Geometry check sheet. Reference: the model listing, model coordinates, mm. Face numbers are marked on the shaded views. A direction names the side the tool comes from. Coordinates: 2 decimals unless noted, no trailing zeros. Write each loop counter-clockwise with the first axis right and the second up, starting at its lowest first coordinate (ties: lowest second). Pieces come first, ordered by that corner, then holes. Notation, with made-up numbers: (56.25, 68) -> (65.25, 68) arc R31 cw to (65.25, 105) -> close; hole circle Ø10 at (74.25, -12.5). An arc over 180 degrees is marked (long way). Answer in a Markdown table with one row per item. Add a question column.
1. Set-up check for the marked faces 1 and 2: record each of +Z, -Z, +X, -X, +Y, -Y from which the full face is reachable in a straight line by a thin tool's end or side.
2. Cross-section at B-B on z = 41. Record the cut outline in (x, y).
3. Scan lines: L1, parallel to Z at x = 3, y = 14; L2, parallel to Z at x = -13, y = -12.5; L3, parallel to Y at x = -4.5, z = 51. Record each from-to range of solid material in increasing order. Write a range as from..to.
4. Mould release check, pull along X, two halves, no side actions. Record for the marked faces 3, 4 and 5: pulls with the +X half, pulls with the -X half, needs draft (parallel to the pull), parting line crosses it, or undercut.
5. Depth check by flat-ended pin: P1, Ø2, axis at y = 11.5, z = 16.5, coming from the -X side; P2, Ø3, axis at x = 3.5, z = 21.5, coming from the +Y side; P3, Ø5, axis at x = 10.5, z = 34.5, coming from the -Y side. Enter the tip coordinate at first touch or a pass-through.
6. Cross-section at C-C on x = 0. Record the cut outline in (y, z), and give its area (3 significant figures).
7. Cross-section at A-A on y = 0. Record the cut outline in (x, z).
8. Cross-section at D-D on z = 4. Record the cut outline in (x, y), and give its area (3 significant figures).
Autodesk Inventor part; units mm, degrees
ref_plane "YZ Plane" through (0, 0, 0) normal (1, 0, 0) x (0, 1, 0)
ref_plane "XZ Plane" through (0, 0, 0) normal (0, 1, 0) x (-1, 0, 0)
ref_plane "XY Plane" through (0, 0, 0) normal (0, 0, 1) x (1, 0, 0)
sketch "Sketch1" plane through (0, 0, 0) normal (0, 0, 1) x (1, 0, 0)
  circle A0 centre (0, 0) radius 14.39
  dimension "d0" = 28.78
extrude "Extrusion1" add sketch "Sketch1" along normal blind 37
sketch "Sketch2" plane through (0, 0, 37) normal (0, 0, 1) x (1, 0, 0)
  circle A0 centre (-5.9617, 0) radius 2.5
  circle A1 centre (5.5337, 0) radius 2.5
  point P0 (0, 0)
  dimension "d3" = 5
  dimension "d4" = 5
extrude "Extrusion2" add sketch "Sketch2" along normal blind 20
sketch "Sketch3" plane through (0, 0, 0) normal (0, 0, -1) x (-1, 0, 0)
  circle A0 centre (0, 0) radius 18.5
  dimension "d7" = 37
extrude "Extrusion3" add sketch "Sketch3" along normal blind 5
sketch "Sketch4" plane through (0, 0, -5) normal (0, 0, -1) x (-1, 0, 0)
  line L0 (-6.8621, 5.2759) -> (7.1379, 5.2759)
  line L1 (7.1379, 5.2759) -> (7.1379, 9.2759)
  line L2 (7.1379, 9.2759) -> (-6.8621, 9.2759)
  line L3 (-6.8621, 9.2759) -> (-6.8621, 5.2759)
  line L4 (-6.8621, 5.2759) -> (7.1379, 9.2759) construction
  line L5 (7.1379, 5.2759) -> (-6.8621, 9.2759) construction
  line L6 (-6.8621, -9.069) -> (7.1379, -9.069)
  line L7 (7.1379, -9.069) -> (7.1379, -5.069)
  line L8 (7.1379, -5.069) -> (-6.8621, -5.069)
  line L9 (-6.8621, -5.069) -> (-6.8621, -9.069)
  line L10 (-6.8621, -9.069) -> (7.1379, -5.069) construction
  line L11 (7.1379, -9.069) -> (-6.8621, -5.069) construction
  point P0 (0, 0)
  point P1 (0.1379, 7.2759)
  point P2 (0.1379, -7.069)
  dimension "d10" = 4
  dimension "d11" = 14
  dimension "d12" = 14
  dimension "d13" = 4
extrude "Extrusion4" cut sketch "Sketch4" against normal blind 2
thread "Thread1"
equation "\"d12\" = d11"
equation "\"d13\" = d10"
properties part number "USB plug"
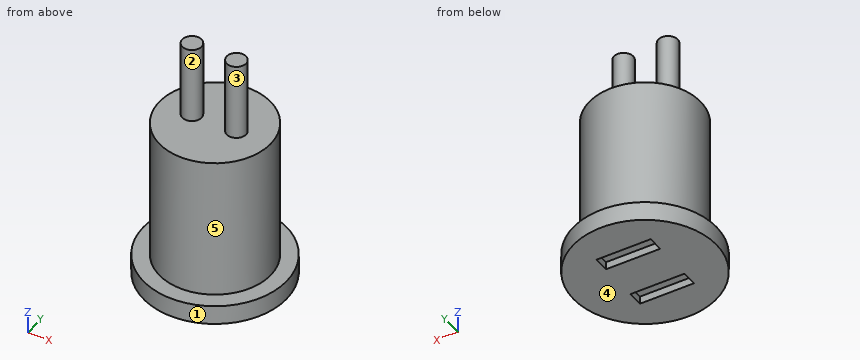
Results found:
| question | item | result |
|---|---|---|
| 1 | face 1 | +Z, -Z |
| 1 | face 2 | +Z |
| 2 | outline | circle Ø5 at (-5.96, 0); circle Ø5 at (5.53, 0) |
| 3 | L1 | z = -5..37 |
| 3 | L2 | z = -5..0 |
| 3 | L3 | y = -2.03..2.03 |
| 4 | face 3 | undercut |
| 4 | face 4 | needs draft |
| 4 | face 5 | parting line crosses it |
| 5 | P1 | stops at x = -9.84 |
| 5 | P2 | stops at y = 14.25 |
| 5 | P3 | stops at y = -11.96 |
| 6 | outline | (-18.5, -5) -> (-9.07, -5) -> (-9.07, -3) -> (-5.07, -3) -> (-5.07, -5) -> (5.28, -5) -> (5.28, -3) -> (9.28, -3) -> (9.28, -5) -> (18.5, -5) -> (18.5, 0) -> (14.39, 0) -> (14.39, 37) -> (-14.39, 37) -> (-14.39, 0) -> (-18.5, 0) -> close |
| 6 | area | 1,230 mm^2 |
| 7 | outline | (-18.5, -5) -> (18.5, -5) -> (18.5, 0) -> (14.39, 0) -> (14.39, 37) -> (8.03, 37) -> (8.03, 57) -> (3.03, 57) -> (3.03, 37) -> (-3.46, 37) -> (-3.46, 57) -> (-8.46, 57) -> (-8.46, 37) -> (-14.39, 37) -> (-14.39, 0) -> (-18.5, 0) -> close |
| 8 | outline | circle Ø28.78 at (0, 0) |
| 8 | area | 651 mm^2 |
